Here's how the part is built. I have some questions about the finished solid (model axes, mm). A direction names the side the tool comes from. Give positions to 0.01 mm unless a question says otherwise; leave off trailing zeros. Loops run counter-clockwise (first coordinate to the right, second up) from the corner with the lowest first, then second, coordinate; pieces in that order, holes last.
Q1. If we section it at A-A (y = 76): Please give me the cut outline in (x, z), plus the area to 3 significant figures.
Q2. We'd pull the mould along Z, two halves only. Please class faces 6 (the face through (-33.917, -3.944, 33.367)), 7 (the face through (212, 214, 0)), 8 (the face through (-22, 217, 0)), 9 (the face through (169, 222, 0)): +Z half, -Z half, draft (parallel to the pull), parting line (faces both ways), or undercut.
Q3. If we section it at C-C (y = 172): Please give me the cut outline in (x, z), plus the area to 3 significant figures.
Q4. Will these pins go through, and if not, where does the flat tip stop? P1, Ø1.5, axis at y = 193, z = -18, coming from the +X side; P2, Ø15, axis at x = 25, y = 206.5, coming from the -Z side; P3, Ø12, axis at y = 100, z = 17.5, coming from the -X side.
Q5. If we section it at D-D (y = 36): Please give me the cut outline in (x, z).
Q6. I need wall thicknesses on line 1 (Y direction, x = -7, z = 0); line 2 (X direction, y = -4.75, z = 42); line 3 (Y direction, x = 14, z = -10.5). Which ranges of each line are inside material? Lowest first, please.
Q7. If we section it at B-B (x = 169): Please give me the cut outline in (y, z).
Q8. For faces 1 (the face through (0, 148, -16)), 2 (the face through (13.5, 211.8, -21)), 3 (the face through (0, 102, 17)), 4 (the face through (-39.635, -3.944, -44.58)), 5 (the face through (169, 200, 0)), which set-ups out of +Z, -Z, +X, -X, +Y, -Y let a thin tool reach every point of the face, with its end or its side?
from build123d import *

# Parameters (mm, degrees)
SKETCH1_W            = 110
SKETCH1_H            = 110
BOSS_EXTRUDE1_DEPTH  = 12
SKETCH2_R            = 9
BOSS_EXTRUDE2_DEPTH  = 8
SKETCH3_R            = 28
BOSS_EXTRUDE3_DEPTH  = 60
SKETCH4_W            = 60
SKETCH4_H            = 52
BOSS_EXTRUDE4_DEPTH  = 25
SKETCH5_W            = 32
SKETCH5_H            = 107
BOSS_EXTRUDE5_DEPTH  = 16
SKETCH6_W            = 72
SKETCH6_H            = 50
BOSS_EXTRUDE6_DEPTH  = 21
SKETCH7_R            = 18
BOSS_EXTRUDE7_DEPTH  = 6
SKETCH8_W            = 115
SKETCH8_H            = 28
BOSS_EXTRUDE8_DEPTH  = 14
SKETCH9_W            = 34
SKETCH9_H            = 44
BOSS_EXTRUDE9_DEPTH  = 17
SKETCH10_R           = 13
BOSS_EXTRUDE10_DEPTH = 15
SKETCH11_W           = 50
SKETCH11_H           = 34
BOSS_EXTRUDE11_DEPTH = 18
SKETCH12_W           = 36
SKETCH12_H           = 18
CUT_EXTRUDE1_DEPTH   = 11
SKETCH13_R           = 6
CUT_EXTRUDE2_DEPTH   = 339.444973371
SKETCH14_R           = 5
CUT_EXTRUDE3_DEPTH   = 339.444973371
SKETCH15_R           = 4
CUT_EXTRUDE4_DEPTH   = 339.444973371
SKETCH16_R           = 3.5
CUT_EXTRUDE5_DEPTH   = 339.444973371


with BuildPart() as part:
    # Sketch1 → Boss-Extrude1 (new body)
    with BuildSketch(Plane(origin=(0, 0, 0), x_dir=(1, 0, 0), z_dir=(0, 1, 0))):
        Rectangle(SKETCH1_W, SKETCH1_H)
    extrude(amount=BOSS_EXTRUDE1_DEPTH)

    # Sketch2 → Boss-Extrude2 (add)
    with BuildSketch(Plane(origin=(0, 0, 0), x_dir=(1, 0, 0), z_dir=(0, 1, 0))):
        with Locations(Location((-40, -40, 0), (0, 0, 270))):
            Circle(SKETCH2_R)
        with Locations(Location((40, -40, 0), (0, 0, 270))):
            Circle(SKETCH2_R)
        with Locations(Location((-40, 40, 0), (0, 0, 270))):
            Circle(SKETCH2_R)
        with Locations(Location((40, 40, 0), (0, 0, 270))):
            Circle(SKETCH2_R)
    extrude(amount=-BOSS_EXTRUDE2_DEPTH)

    # Sketch3 → Boss-Extrude3 (add)
    with BuildSketch(Plane(origin=(0, 0, 0), x_dir=(1, 0, 0), z_dir=(0, 1, 0))):
        with Locations(Location((0, 0, 0), (0, 0, 90))):
            Circle(SKETCH3_R)
    extrude(amount=BOSS_EXTRUDE3_DEPTH)

    # Sketch4 → Boss-Extrude4 (add, symmetric)
    with BuildSketch(Plane.XY):
        with Locations((0, 76)):
            Rectangle(SKETCH4_W, SKETCH4_H)
    extrude(amount=BOSS_EXTRUDE4_DEPTH, both=True)

    # Sketch5 → Boss-Extrude5 (add, symmetric)
    with BuildSketch(Plane.XY):
        with Locations((0, 151.5)):
            Rectangle(SKETCH5_W, SKETCH5_H)
    extrude(amount=BOSS_EXTRUDE5_DEPTH, both=True)

    # Sketch6 → Boss-Extrude6 (add, symmetric)
    with BuildSketch(Plane.XY):
        with Locations((14, 217)):
            Rectangle(SKETCH6_W, SKETCH6_H)
    extrude(amount=BOSS_EXTRUDE6_DEPTH, both=True)

    # Sketch7 → Boss-Extrude7 (add, symmetric)
    with BuildSketch(Plane.XY):
        with Locations((14, 217)):
            Circle(SKETCH7_R)
    extrude(amount=BOSS_EXTRUDE7_DEPTH, both=True)

    # Sketch8 → Boss-Extrude8 (add, symmetric)
    with BuildSketch(Plane.XY):
        with Locations((102.5, 222)):
            Rectangle(SKETCH8_W, SKETCH8_H)
    extrude(amount=BOSS_EXTRUDE8_DEPTH, both=True)

    # Sketch9 → Boss-Extrude9 (add, symmetric)
    with BuildSketch(Plane.XY):
        with Locations((169, 222)):
            Rectangle(SKETCH9_W, SKETCH9_H)
    extrude(amount=BOSS_EXTRUDE9_DEPTH, both=True)

    # Sketch10 → Boss-Extrude10 (add, symmetric)
    with BuildSketch(Plane.XY):
        with Locations((186, 222)):
            Circle(SKETCH10_R)
    extrude(amount=BOSS_EXTRUDE10_DEPTH, both=True)

    # Sketch11 → Boss-Extrude11 (add, symmetric)
    with BuildSketch(Plane.XY):
        with Locations((203, 223)):
            Rectangle(SKETCH11_W, SKETCH11_H)
    extrude(amount=BOSS_EXTRUDE11_DEPTH, both=True)

    # Sketch12 → Cut-Extrude1 (cut, symmetric)
    with BuildSketch(Plane.XY):
        with Locations((214, 223)):
            Rectangle(SKETCH12_W, SKETCH12_H)
    extrude(amount=CUT_EXTRUDE1_DEPTH, both=True, mode=Mode.SUBTRACT)

    # Sketch13 → Cut-Extrude2 (cut, through all)
    with BuildSketch(Plane(origin=(0, 0, 0), x_dir=(0, 0, -1), z_dir=(1, 0, 0))):
        with Locations((0, 76)):
            Circle(SKETCH13_R)
    extrude(amount=-CUT_EXTRUDE2_DEPTH, mode=Mode.SUBTRACT)

    # Sketch14 → Cut-Extrude3 (cut, through all)
    with BuildSketch(Plane.XY):
        with Locations((14, 217)):
            Circle(SKETCH14_R)
    extrude(amount=-CUT_EXTRUDE3_DEPTH, mode=Mode.SUBTRACT)

    # Sketch15 → Cut-Extrude4 (cut, through all)
    with BuildSketch(Plane.XY):
        with Locations((169, 222)):
            Circle(SKETCH15_R)
    extrude(amount=-CUT_EXTRUDE4_DEPTH, mode=Mode.SUBTRACT)

    # Sketch16 → Cut-Extrude5 (cut, through all)
    with BuildSketch(Plane(origin=(0, 0, 0), x_dir=(1, 0, 0), z_dir=(0, 1, 0))):
        with Locations(Location((-42, -42, 0), (0, 0, 270))):
            Circle(SKETCH16_R)
        with Locations(Location((42, -42, 0), (0, 0, 270))):
            Circle(SKETCH16_R)
        with Locations(Location((-42, 42, 0), (0, 0, 270))):
            Circle(SKETCH16_R)
        with Locations(Location((42, 42, 0), (0, 0, 270))):
            Circle(SKETCH16_R)
    extrude(amount=-CUT_EXTRUDE5_DEPTH, mode=Mode.SUBTRACT)


solid = part.part
Check sheet entries:
1. outline: (-30, -25) - (30, -25) - (30, 25) - (-30, 25) - (-30, 6) - (0, 6) - (0, -6) - (-30, -6) - close
1. area: 2,640 mm2
2. face 6: undercut
2. face 7: undercut
2. face 8: draft
2. face 9: -Z half
3. outline: (-16, -16) - (16, -16) - (16, 16) - (-16, 16) - close
3. area: 1,020 mm2
4. P1: stops at x = 50
4. P2: stops at z = -21
4. P3: stops at x = -30
5. outline: circle Ø56 at (0, 0)
6. line 1: y = 0 to 70, 82 to 242
6. line 2: x = -48.77 to -45.5, -38.5 to -31.23, 31.23 to 38.5, 45.5 to 48.77
6. line 3: y = 0 to 212, 222 to 242
7. outline: (200, -17) - (218, -17) - (218, 0) - (226, 0) - (226, -17) - (244, -17) - (244, 17) - (200, 17) - close
8. face 1: -Z, +X, -X
8. face 2: -Z, +X, -X, +Y
8. face 3: none
8. face 4: -Y
8. face 5: +Z, -Z, +X, -Y
